Autodesk Inventor part; units mm, degrees
ref_plane "XZ Plane" through (0, 0, 0) normal (0, 1, 0) x (-1, 0, 0)
ref_plane "XY Plane" through (0, 0, 0) normal (0, 0, 1) x (1, 0, 0)
sketch "Sketch1" plane through (0, 0, 0) normal (0, 0, 1) x (1, 0, 0)
  line L0 (-12.7, -25.4) -> (12.7, -25.4)
  line L1 (12.7, -25.4) -> (12.7, 25.4)
  line L2 (12.7, 25.4) -> (-12.7, 25.4)
  line L3 (-12.7, 25.4) -> (-12.7, -25.4)
  line L4 (-12.7, -25.4) -> (12.7, 25.4) construction
  line L5 (12.7, -25.4) -> (-12.7, 25.4) construction
  line L6 (-9.525, 22.225) -> (9.525, 22.225)
  line L7 (9.525, 22.225) -> (9.525, -22.225)
  line L8 (9.525, -22.225) -> (-9.525, -22.225)
  line L9 (-9.525, -22.225) -> (-9.525, 22.225)
  point P0 (0, 0)
  dimension "width" = 25.4
  dimension "height" = 50.8
  dimension "thickness" = 3.175
extrude "Extrusion1" add sketch "Sketch1" along normal mid plane 254
sketch "Sketch2" plane through (12.7, -25.4, 127) normal (1, 0, 0) x (0, 0, -1)
  line L0 (254, 50.8) -> (254, 0) construction
  line L1 (254, 0) -> (0, 0) construction
  line L2 (0, 0) -> (0, 50.8) construction
  line L3 (0, 50.8) -> (254, 50.8) construction
  circle A0 centre (31.75, 25.4) radius 23.8125 construction
  circle A1 centre (31.75, 25.4) radius 25.4 construction
  point P0 (127, 25.4)
  point P1 (57.15, 25.4)
  point P2 (53.747, 38.1)
  point P3 (44.45, 47.397)
  point P4 (31.75, 50.8)
  point P5 (19.05, 47.397)
  point P6 (9.753, 38.1)
  point P7 (6.35, 25.4)
  point P8 (9.753, 12.7)
  point P9 (19.05, 3.403)
  point P10 (31.75, 0)
  point P11 (44.45, 3.403)
  point P12 (53.747, 12.7)
  point P13 (55.5625, 25.4)
  point P14 (43.6562, 46.0222)
  point P15 (19.8437, 46.0222)
  point P16 (7.9375, 25.4)
  point P17 (19.8437, 4.7778)
  point P18 (43.6562, 4.7778)
  dimension "d13" = 47.625
  dimension "d14" = 50.8
  dimension "d5" = 31.75
  dimension "d17" = 360
  dimension "d21" = 360
hole "Hole1" at (12.7, 0, 95.25) direction (-1, 0, 0) diameter 28.956 end through all
hole "Hole2" at (12.7, 12.7, 73.253) at (12.7, 0, 69.85) at (12.7, -12.7, 73.253) at (12.7, -12.7, 117.247) at (12.7, 0, 120.65) at (12.7, 12.7, 117.247) direction (-1, 0, 0) diameter 5.1054 end through all
hole "Hole3" at (12.7, -20.6222, 107.1562) at (12.7, -20.6222, 83.3438) at (12.7, 0, 119.0625) at (12.7, 20.6222, 107.1562) at (12.7, 20.6222, 83.3438) at (12.7, 0, 71.4375) direction (-1, 0, 0) diameter 4.4958 end through all
properties part number "CL4-002" material "Aluminum 6061"
Source: CAD feature listing. Evaluate the final solid. Frame: model axes, mm. A direction names the side the tool comes from. Give positions to 0.01 mm unless a question says otherwise; leave off trailing zeros. Order: outer loops, then holes, each group sorted by start corner. A loop starts at its lowest first (then second) coordinate and runs counter-clockwise, first axis right, second up. Notation, with made-up numbers: (-27, 48.5) -> (4, 48.5) arc R23 ccw to (4, 87.5) -> close; hole circle Ø6 at (43.25, 7.5). An arc over 180 degrees is marked (long way). Use a Markdown table: item, result.
Q1. Pull-direction query (Y, two-part tool) for faces 3 (the face through (0, -25.4, -2)), 4 (the face through (12.7, 0, -2)), 5 (the face through (11.09, -4.35, 81.44)); classes: +Y half, -Y half, draft (parallel to the pull), parting line (faces both ways), or undercut.
A:
| item | result |
|---|---|
| face 3 | -Y half |
| face 4 | draft |
| face 5 | undercut |
Q2. Section A-A (y = 0). State how many separate pieces and enclosed holes the cut face has, and give its area (3 significant figures).
A:
| item | result |
|---|---|
| separate pieces | 8 |
| enclosed holes | 0 |
| area | 1,350 mm^2 |
Q3. First-contact query: P1, Ø3.5, axis at y = 0, z = 119.06, coming from the +X side. Flat tip, straight axial feed; report the tip coordinate or a pass-through.
A:
| item | result |
|---|---|
| P1 | through |
Q4. Material intervals for line 1 (X direction, y = 21, z = 53) (3 decimals); line 2 (Y direction, x = 0.75, z = 7) (3 decimals); line 3 (Z direction, x = -10, y = 11), sorted ascending. Write a range as [from, to].
A:
| item | result |
|---|---|
| line 1 | [-12.7, -9.525], [9.525, 12.7] |
| line 2 | [-25.4, -22.225], [22.225, 25.4] |
| line 3 | [-127, 71.35], [75.16, 85.84], [104.66, 115.34], [119.15, 127] |
Q5. Section B-B (z = -91.5). Return the cut outline in (x, y) (3 decimals), and give its area (3 significant figures).
A:
| item | result |
|---|---|
| outline | (-12.7, -25.4) -> (12.7, -25.4) -> (12.7, 25.4) -> (-12.7, 25.4) -> close; hole (-9.525, -22.225) -> (9.525, -22.225) -> (9.525, 22.225) -> (-9.525, 22.225) -> close |
| area | 444 mm^2 |
Q6. Section D-D (z = 95.25). Return the cut outline in (x, y) (3 decimals).
A:
| item | result |
|---|---|
| outline | (-12.7, -25.4) -> (12.7, -25.4) -> (12.7, -14.478) -> (9.525, -14.478) -> (9.525, -22.225) -> (-9.525, -22.225) -> (-9.525, -14.478) -> (-12.7, -14.478) -> close; (-12.7, 14.478) -> (-9.525, 14.478) -> (-9.525, 22.225) -> (9.525, 22.225) -> (9.525, 14.478) -> (12.7, 14.478) -> (12.7, 25.4) -> (-12.7, 25.4) -> close |
Q7. Section C-C (x = 0.75). Return the cut outline in (y, z) (3 decimals).
A:
| item | result |
|---|---|
| outline | (-25.4, -127) -> (-22.225, -127) -> (-22.225, 81.768) arc R2.248 cw to (-22.225, 84.92) -> (-22.225, 105.58) arc R2.248 cw to (-22.225, 108.732) -> (-22.225, 127) -> (-25.4, 127) -> close; (22.225, -127) -> (25.4, -127) -> (25.4, 127) -> (22.225, 127) -> (22.225, 108.732) arc R2.248 cw to (22.225, 105.58) -> (22.225, 84.92) arc R2.248 cw to (22.225, 81.768) -> close |
Q8. Access query for faces 1 (the face through (11.1, 13.7, 114.9)), 2 (the face through (0, 22.225, 95)). Directions: +Z, -Z, +X, -X, +Y, -Y. A direction counts if a zero-diameter tool reaches every point of the face in a straight line with its end or side. Return the directions, or none.
A:
| item | result |
|---|---|
| face 1 | +X, -X |
| face 2 | +Z, -Z |
